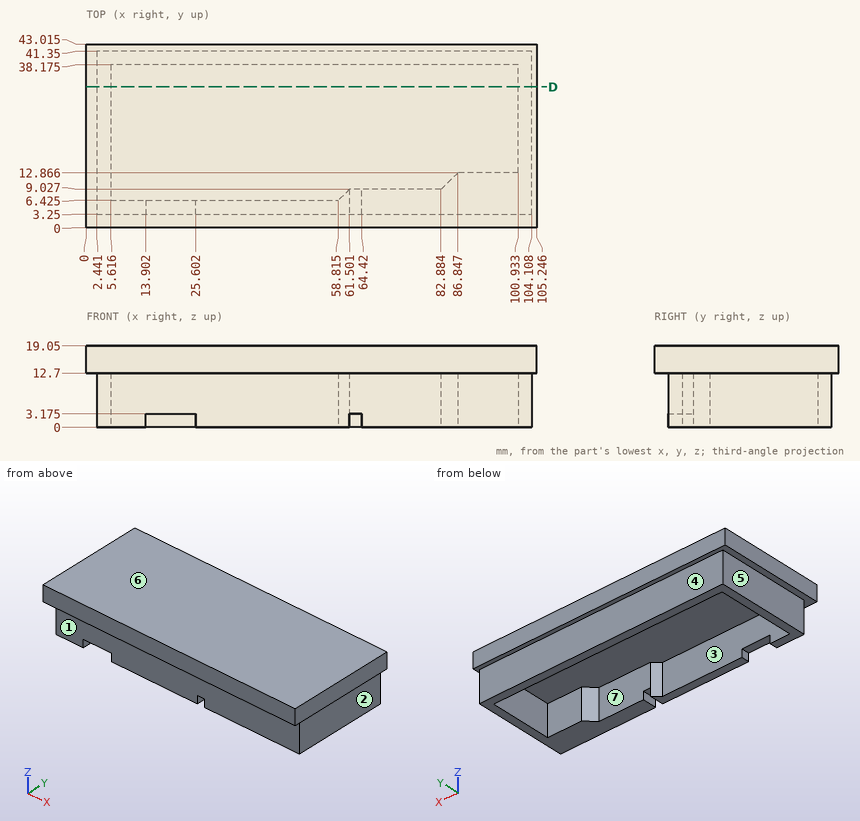
Study the drawing (mm; zero at the part's minimum x, y, z) and answer. A direction names the side the tool comes from. Give positions to 0.01 mm unless a question says otherwise; leave off trailing zeros. Write each loop counter-clockwise with the first axis right and the second up, starting at its lowest first coordinate (ties: lowest second). Pieces come first, ordered by that corner, then holes. Notation, with made-up numbers: (-39, 12) - (2, 12) arc R29 ccw to (2, 41) - close; hole circle Ø1 at (-21, -8.75). An arc over 180 degrees is marked (long way). One line per question, with ' | ' between items. Start each with the question number.
1. Determine the mould class of the marked faces 5, 6 and 7 for opening direction X: +X half, -X half, draft (parallel to the pull), parting line (faces both ways), or undercut.
2. For the marked faces 1, 2, 3 and 4, determine the directions among +Z, -Z, +X, -X, +Y, -Y from which every point of the face is accessible in a straight line to the end or side of a thin tool.
3. Straight lines are drawn through the part: line 1 (X direction, y = 36, z = 9.75); line 2 (Z direction, x = 16, y = 13); line 3 (Y direction, x = 5, z = 7.75). For each, find the intervals that lie inside material, in ascending order.
4. Given P1, Ø4, axis at x = 97, z = 6, coming from the +Y side; P2, Ø10, axis at x = 67.5, z = 5.5, coming from the -Y side; P3, Ø3.5, axis at y = 7.5, z = 2.5, coming from the +X side, each flat-ended and moving along its own axis, determine where each tip first touches the part or whether it passes through.
5. Section D-D, the plane y = 33 is taken. Determine the outline of the cut face in (x, z).
Result:
1) face 5: -X half | face 6: draft | face 7: undercut
2) face 1: -Z, +X, -X, -Y | face 2: -Z, +X, +Y, -Y | face 3: -Z | face 4: -Z, +X, -X, +Y
3) line 1: x = 2.44 to 5.62, 100.93 to 104.11 | line 2: z = 12.7 to 19.05 | line 3: y = 3.25 to 41.35
4) P1: stops at y = 41.35 | P2: stops at y = 3.25 | P3: stops at x = 104.11
5) outline: (0, 12.7) - (2.44, 12.7) - (2.44, 0) - (5.62, 0) - (5.62, 12.7) - (100.93, 12.7) - (100.93, 0) - (104.11, 0) - (104.11, 12.7) - (105.25, 12.7) - (105.25, 19.05) - (0, 19.05) - close
